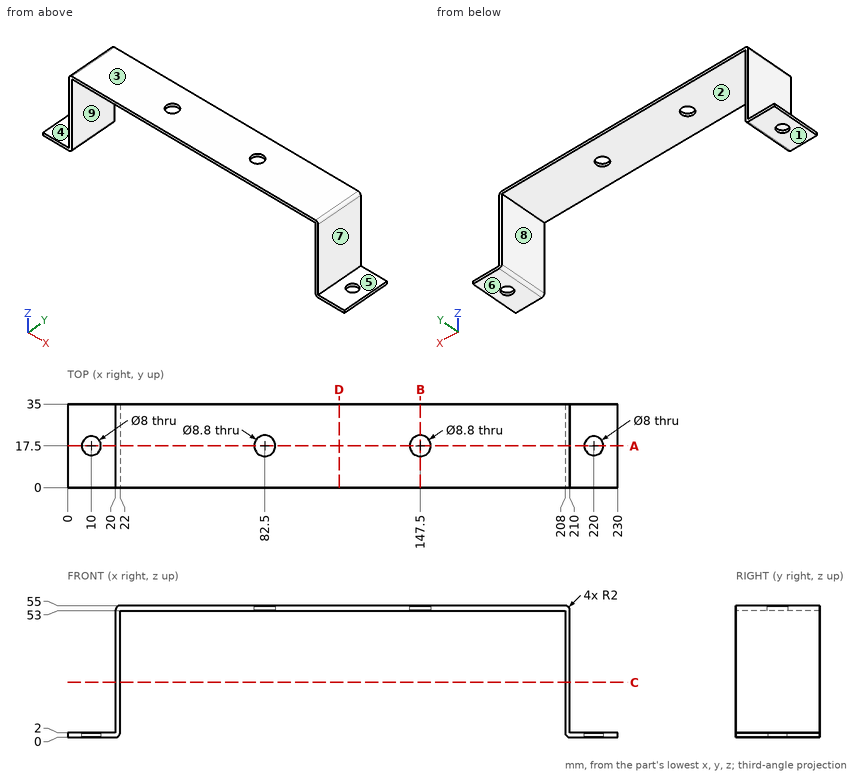
Check sheet for the drawn part. Datum: minimum x, y, z corner. Units: mm. A direction names the side the tool comes from. Give positions to 0.01 mm unless a question says otherwise; leave off trailing zeros. Write each loop counter-clockwise with the first axis right and the second up, starting at its lowest first coordinate (ties: lowest second). Pieces come first, ordered by that corner, then holes.
(1) Cross-section at C-C (z = 23). Enter the section's corners in (x, y), plus the area to 3 significant figures.
(2) Gauge pin test, flat ends, axial feed: pin 1 (1 mm diameter, centred on y = 28, z = 31, fed in from +X); pin 2 (5 mm diameter, centred on y = 20, z = 31, fed in from -X); pin 3 (9 mm diameter, centred on x = 220, y = 17.5, fed in from +Z). Record the tip position at first contact, or that the pin passes through.
(3) Mould release check, pull along X, two halves, no side actions. Record for the marked faces 6, 7, 8 and 9: +X half, -X half, draft (parallel to the pull), parting line (faces both ways), or undercut.
(4) Cross-section at A-A (y = 17.5). State how many separate pieces and enclosed holes the cut face has, plus the area to 3 significant figures.
(5) Material ranges on line 1 (X direction, y = 30, z = 41); line 2 (Y direction, x = 10, z = 1.45); line 3 (Z direction, x = 135, y = 30.5), recorded low to high.
(6) Access from +Z, -Z, +X, -X, +Y, -Y to the whole of each face (thin tool, end or side, straight path). Record for the marked faces 1, 2, 3, 4 and 5.
(7) Cross-section at B-B (x = 147.5). Enter the section's corners in (y, z), plus the area to 3 significant figures.
(8) Cross-section at D-D (x = 113.5). Enter the section's corners in (y, z), plus the area to 3 significant figures.
Worked out:
1. outline: (20, 0) - (22, 0) - (22, 35) - (20, 35) - close; (208, 0) - (210, 0) - (210, 35) - (208, 35) - close
1. area: 140 mm2
2. pin 1: stops at x = 210
2. pin 2: stops at x = 20
2. pin 3: stops at z = 2
3. face 6: draft
3. face 7: +X half
3. face 8: undercut
3. face 9: undercut
4. separate pieces: 5
4. enclosed holes: 0
4. area: 601 mm2
5. line 1: x = 20 to 22, 208 to 210
5. line 2: y = 0 to 13.5, 21.5 to 35
5. line 3: z = 53 to 55
6. face 1: -Z, +X, -X, +Y, -Y
6. face 2: -Z, +Y, -Y
6. face 3: +Z, +X, -X, +Y, -Y
6. face 4: +Z, -X, +Y, -Y
6. face 5: +Z, +X, +Y, -Y
7. outline: (0, 53) - (13.1, 53) - (13.1, 55) - (0, 55) - close; (21.9, 53) - (35, 53) - (35, 55) - (21.9, 55) - close
7. area: 52.4 mm2
8. outline: (0, 53) - (35, 53) - (35, 55) - (0, 55) - close
8. area: 70.0 mm2
